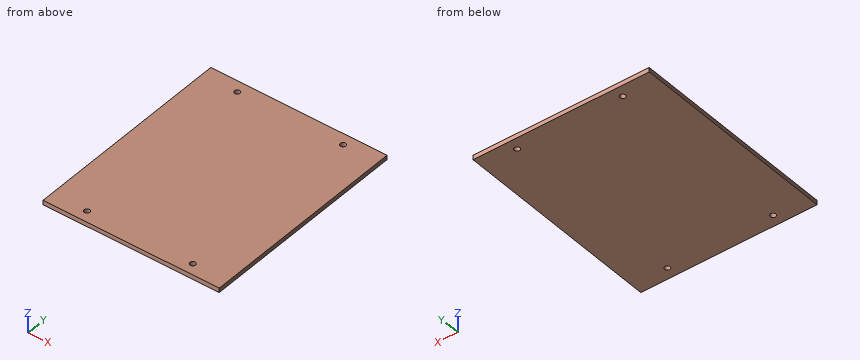
```python
from build123d import *

# Parameters (mm, degrees)
F0_W     = 254
F0_H     = 304.8
F1_DEPTH = 6.35
F3_D     = 7.9248
F4_D     = 7.9248
F5_D     = 7.9248
F6_D     = 7.9248


with BuildPart() as f1:
    # F0 (on Top) → F1 (new body)
    with BuildSketch(Plane.XY):
        with Locations((127, 152.4)):
            Rectangle(F0_W, F0_H)
    extrude(amount=-F1_DEPTH)

    # F3 (through all)
    with Locations(Plane.XY):
        with Locations((50.8, 288.925)):
            Hole(F3_D / 2)

    # F4 (through all)
    with Locations(Plane.XY):
        with Locations((203.2, 288.925)):
            Hole(F4_D / 2)

    # F5 (through all)
    with Locations(Plane.XY):
        with Locations((203.2, 15.875)):
            Hole(F5_D / 2)

    # F6 (through all)
    with Locations(Plane.XY):
        with Locations((50.8, 15.875)):
            Hole(F6_D / 2)


solid = f1.part
```
The model under review builds one solid part; all positions refer to its coordinate system, in mm. Give positions to 0.01 mm unless a question says otherwise; leave off trailing zeros. Write each loop counter-clockwise with the first axis right and the second up, starting at its lowest first coordinate (ties: lowest second). Pieces come first, ordered by that corner, then holes. Notation, with made-up numbers: M 42,27 L 55,27 A11 ccw 55,31 Z; hole C 71.25,58 d9. An arc over 180 degrees is marked long. Write each question's results on one line, items separated by ' | '. Start each with the question number.
1. We need section A-A (x = 203.2). Write out the cut boundary in (y, z), and give its area (3 significant figures).
2. For probe 1 along Y at (x, z) = (203.2, -1.5); probe 2 along Y at (x, z) = (205.5, -2.25); probe 3 along X at (y, z) = (15, -5), list the stretches that pass through material, from the lowest coordinate up. Write a range as [from, to].
3. Insertion check: pin 1 Ø6.5 at (x, y) = (50.8, 15.875) entering from +Z; pin 2 Ø8 at (x, y) = (32.5, 158) entering from +Z. Each pin has a flat end and moves straight along its axis. Give the tip position at first contact, or say it passes through.
Results found:
1) outline: M 0,-6.35 L 11.91,-6.35 L 11.91,0 L 0,0 Z; M 19.84,-6.35 L 284.96,-6.35 L 284.96,0 L 19.84,0 Z; M 292.89,-6.35 L 304.8,-6.35 L 304.8,0 L 292.89,0 Z | area: 1,830 mm^2
2) probe 1: y = [0, 11.91], [19.84, 284.96], [292.89, 304.8] | probe 2: y = [0, 12.65], [19.1, 285.7], [292.15, 304.8] | probe 3: x = [0, 46.94], [54.66, 199.34], [207.06, 254]
3) pin 1: passes through | pin 2: stops at z = 0
